```python
from build123d import *

# Parameters (mm, degrees)
F0_R     = 0.5
F1_DEPTH = 7.6
F2_R     = 1
F2_R_2   = 0.5
F3_DEPTH = 2.8


with BuildPart() as f1:
    # F0 (on Top) → F1 (new body)
    with BuildSketch(Plane.XY):
        Circle(F0_R)
    extrude(amount=F1_DEPTH)

    # F2 (on face) → F3 (join)
    with BuildSketch(Plane.XY.offset(7.6)):
        Circle(F2_R)
        Circle(F2_R_2, mode=Mode.SUBTRACT)
        Circle(F2_R_2)
    extrude(amount=F3_DEPTH)

    # F4 (on Front) → F5 (revolve)
    with BuildSketch(Plane.XZ):
        with BuildLine():
            Line((0, 10.4), (1, 10.4))
            ThreePointArc((1, 10.4), (0.707107, 11.107107), (0, 11.4))
            Line((0, 11.4), (0, 10.4))
        make_face()
    revolve(axis=Axis((0, 0, 7.5), (0, 0, 1)))


solid = f1.part
```
The listing builds one solid part. Answer for the finished solid, in the listing's coordinates (mm). A direction names the side the tool comes from. Give positions to 0.01 mm unless a question says otherwise; leave off trailing zeros. Loops run counter-clockwise (first coordinate to the right, second up) from the corner with the lowest first, then second, coordinate; pieces in that order, holes last. Notation, with made-up numbers: M -20.75,59.25 L 14.25,59.25 A11 ccw 14.25,80.25 Z; hole C 44.25,32.25 d10. An arc over 180 degrees is marked long. One line per item, written item: value.
1. For faces 1 (the face through (0, -1, 9)), 2 (the face through (-0.108, -0.488, 3.747)), determine the directions among +Z, -Z, +X, -X, +Y, -Y from which every point of the face is accessible in a straight line to the end or side of a thin tool.
Found:
face 1: +Z, -Z
face 2: -Z
2. Section A-A on z = 5 is taken. Determine the outline of the cut face in (x, y).
Found:
outline: C 0,0 d1
3. Find the intervals of material crossed by probe 1 along X at (y, z) = (-0.15, 5.5); probe 2 along Z at (x, y) = (0.35, 0.85); probe 3 along Z at (x, y) = (0.35, 0.2), in increasing order.
Found:
probe 1: -0.48 to 0.48
probe 2: 7.6 to 10.79
probe 3: 0 to 11.32
4. Section B-B on z = 8 is taken. Determine the outline of the cut face in (x, y).
Found:
outline: C 0,0 d2
